Read the model definition and answer for the solid it produces. Units are mm, in the model's axes. A direction names the side the tool comes from. Coordinates: 2 decimals unless noted, no trailing zeros. Write each loop counter-clockwise with the first axis right and the second up, starting at its lowest first coordinate (ties: lowest second). Pieces come first, ordered by that corner, then holes.
1) The part is cut by section A-A (z = 122.25). Determine the outline of the cut face in (x, y), then the cut area to 3 significant figures.
2) The part is cut by section C-C (x = 138). Determine the outline of the cut face in (y, z), then the cut area to 3 significant figures.
3) Which of the six approach directions +Z, -Z, +X, -X, +Y, -Y give full straight-line access (tool end or side, diameter ignored) to faces 1 (the face through (63, 9.05, 2)), 2 (the face through (153, 13, 78)), 3 (the face through (45.548, 3.131, 40.268))?
4) Find the intervals of material crossed by line 1 (X direction, y = 4.25, z = 179.5); line 2 (Z direction, x = 43, y = 3.25); line 3 (Z direction, x = 138, y = 4.5), in increasing order.
5) The part is cut by section B-B (x = 18.5). Determine the outline of the cut face in (y, z), then the cut area to 3 significant figures.
6) The part is cut by section D-D (x = 43). Determine the outline of the cut face in (y, z), then the cut area to 3 significant figures.
7) Determine the mould class of faces 4 (the face through (129, 17, 2)), 5 (the face through (58.988, 3.219, 177.304)), 6 (the face through (117, 9, 158.5)) for opening direction Z: +Z half, -Z half, draft (parallel to the pull), parting line (faces both ways), or undercut.
8) Each of these flat-tipped pins is pushed along its axis until it touches: pin 1 Ø1 at (x, y) = (27, 13) entering from -Z; pin 2 Ø4.5 at (x, z) = (43, 122.25) entering from +Y; pin 3 Ø6.5 at (x, z) = (93, 122.25) entering from -Y; pin 4 Ø1.5 at (x, z) = (61, 2.5) entering from +Y. Where does it stop, or does it pass through?
from build123d import *

# Parameters (mm, degrees)
SKETCH1_W                      = 158
SKETCH1_H                      = 199.5
BOSS_EXTRUDE1_DEPTH            = 6.35
SKETCH2_W                      = 81
SKETCH2_H                      = 41
CUT_EXTRUDE1_DEPTH             = 7.35
BOSS_EXTRUDE2_DEPTH            = 12.7
M4_CLEARANCE_HOLE1_D           = 4.5
M4_CLEARANCE_HOLE1_DEPTH       = 6.35
CUT_EXTRUDE2_REACH             = 201.5
SKETCH7_W                      = 129
SKETCH7_H                      = 10
FILLET1_R                      = 5
F_5_1_5_1_DIAMETER_HOLE1_D     = 5.1
F_5_1_5_1_DIAMETER_HOLE1_DEPTH = 6.35


with BuildPart() as part:
    # Sketch1 → Boss-Extrude1 (new body)
    with BuildSketch(Plane(origin=(0, 0, 0), x_dir=(1, 0, 0), z_dir=(0, 1, 0))):
        with Locations((79, -99.75)):
            Rectangle(SKETCH1_W, SKETCH1_H)
    extrude(amount=BOSS_EXTRUDE1_DEPTH)

    # Sketch2 → Cut-Extrude1 (cut, through all)
    with BuildSketch(Plane(origin=(0, 6.35, 0), x_dir=(1, 0, 0), z_dir=(0, 1, 0))):
        with Locations((117.5, -179)):
            Rectangle(SKETCH2_W, SKETCH2_H)
    extrude(amount=-CUT_EXTRUDE1_DEPTH, mode=Mode.SUBTRACT)

    # Sketch3 → Boss-Extrude2 (add)
    with BuildSketch(Plane(origin=(0, 6.35, 0), x_dir=(1, 0, 0), z_dir=(0, 1, 0))):
        Polygon((0, 0), (0, -5), (153, -5), (153, -153.5), (72, -153.5), (72, -194.5), (0, -194.5), (0, -199.5), (72, -199.5), (77, -199.5), (77, -158.5), (158, -158.5), (158, 0), align=None)
    extrude(amount=BOSS_EXTRUDE2_DEPTH)

    # M4 Clearance Hole1
    with Locations(Plane.XZ):
        with Locations((138, 54.25), (18.5, 179.5), (58.5, 179.5), (138, 129.25), (138, 104.25), (138, 29.25)):
            Hole(M4_CLEARANCE_HOLE1_D / 2, depth=M4_CLEARANCE_HOLE1_DEPTH)

    # Sketch7 → Cut-Extrude2 (cut, up to next)
    with BuildSketch(Plane(origin=(0, 0, 0), x_dir=(-1, 0, 0), z_dir=(0, 0, -1)), mode=Mode.PRIVATE) as cut_extrude2_sk1:
        with Locations((-64.5, 14.05)):
            Rectangle(SKETCH7_W, SKETCH7_H)
    cut_extrude2_tool1 = extrude(cut_extrude2_sk1.sketch, amount=-CUT_EXTRUDE2_REACH, mode=Mode.PRIVATE) & part.part
    add(cut_extrude2_tool1.solids().sort_by_distance((64.5, 14.05, 0))[0], mode=Mode.SUBTRACT)

    # Fillet1
    fillet1_edges = [part.edges().sort_by_distance(p)[0] for p in [
        (129, 9.05, 2.5),
    ]]
    fillet(fillet1_edges, radius=FILLET1_R)

    # Ø5.1 (5.1) Diameter Hole1
    with Locations(Plane(origin=(0, 6.35, 0), x_dir=(1, 0, 0), z_dir=(0, 1, 0))):
        with Locations((43, -40.38), (43, -122.25), (93, -122.25), (93, -40.38)):
            Hole(F_5_1_5_1_DIAMETER_HOLE1_D / 2, depth=F_5_1_5_1_DIAMETER_HOLE1_DEPTH)


solid = part.part
Reported:
1. outline: (0, 0) - (40.45, 0) - (40.45, 6.35) - (0, 6.35) - close; (45.55, 0) - (90.45, 0) - (90.45, 6.35) - (45.55, 6.35) - close; (95.55, 0) - (158, 0) - (158, 19.05) - (153, 19.05) - (153, 6.35) - (95.55, 6.35) - close
1. area: 1,000 mm2
2. outline: (0, 0) - (19.05, 0) - (19.05, 5) - (6.35, 5) - (6.35, 27) - (0, 27) - close; (0, 31.5) - (6.35, 31.5) - (6.35, 52) - (0, 52) - close; (0, 56.5) - (6.35, 56.5) - (6.35, 102) - (0, 102) - close; (0, 106.5) - (6.35, 106.5) - (6.35, 127) - (0, 127) - close; (0, 131.5) - (6.35, 131.5) - (6.35, 153.5) - (19.05, 153.5) - (19.05, 158.5) - (0, 158.5) - close
2. area: 1,020 mm2
3. face 1: -Z, -X, +Y
3. face 2: -X, +Y
3. face 3: +Y, -Y
4. line 1: x = 0 to 16.25, 20.75 to 56.25, 60.75 to 77
4. line 2: z = 0 to 37.83, 42.93 to 119.7, 124.8 to 199.5
4. line 3: z = 0 to 27, 31.5 to 52, 56.5 to 102, 106.5 to 127, 131.5 to 158.5
5. outline: (0, 0) - (9.05, 0) - (9.05, 5) - (6.35, 5) - (6.35, 177.25) - (0, 177.25) - close; (0, 181.75) - (6.35, 181.75) - (6.35, 194.5) - (19.05, 194.5) - (19.05, 199.5) - (0, 199.5) - close
5. area: 1,320 mm2
6. outline: (0, 0) - (9.05, 0) - (9.05, 5) - (6.35, 5) - (6.35, 37.83) - (0, 37.83) - close; (0, 42.93) - (6.35, 42.93) - (6.35, 119.7) - (0, 119.7) - close; (0, 124.8) - (6.35, 124.8) - (6.35, 194.5) - (19.05, 194.5) - (19.05, 199.5) - (0, 199.5) - close
6. area: 1,280 mm2
7. face 4: draft
7. face 5: undercut
7. face 6: +Z half
8. pin 1: stops at z = 194.5
8. pin 2: passes through
8. pin 3: stops at y = 0
8. pin 4: stops at y = 9.05
